```python
from build123d import *

# Parameters (mm, degrees)
SKETCH1_R           = 1.175
BOSS_EXTRUDE1_DEPTH = 6.4
BOSS_EXTRUDE2_DEPTH = 3.2
SKETCH4_W           = 0.5
SKETCH4_H           = 3.9
BOSS_EXTRUDE3_DEPTH = 3.2
SKETCH5_R           = 0.8
CUT_EXTRUDE1_DEPTH  = 22.246411462


with BuildPart() as part:
    # Sketch1 → Boss-Extrude1 (new body)
    with BuildSketch(Plane(origin=(0, 0, 0), x_dir=(1, 0, 0), z_dir=(0, 1, 0))):
        Polygon((-10.95, -2.5), (-10.75, -2.7), (-8.25, -2.7), (-8.05, -2.5), (-1.45, -2.5), (-1.25, -2.7), (1.25, -2.7), (1.45, -2.5), (5.2, -2.5), (5.2, 7), (-4.7, 7), (-5.4, 7.7), (-14.6, 7.7), (-14.6, -2.5), align=None)
        with Locations(Location((0, 0, 0), (0, 0, 270))):
            Circle(SKETCH1_R, mode=Mode.SUBTRACT)
        with Locations(Location((-9.5, 0, 0), (0, 0, 270))):
            Circle(SKETCH1_R, mode=Mode.SUBTRACT)
    extrude(amount=BOSS_EXTRUDE1_DEPTH)

    # Sketch3 → Boss-Extrude2 (add)
    with BuildSketch(Plane(origin=(0, 1.6, 0), x_dir=(1, 0, 0), z_dir=(0, 1, 0))):
        with BuildLine():
            Line((-8.5, 7), (-6.5, 7))
            Line((-6.5, 7), (-6.5, 7.9))
            ThreePointArc((-6.5, 7.9), (-7.5, 8.9), (-8.5, 7.9))
            Line((-8.5, 7.9), (-8.5, 7))
        make_face()
    extrude(amount=BOSS_EXTRUDE2_DEPTH)

    # Sketch4 → Boss-Extrude3 (add)
    with BuildSketch(Plane(origin=(0, 1.6, 0), x_dir=(1, 0, 0), z_dir=(0, 1, 0))):
        with Locations((-12.75, -4.45)):
            Rectangle(SKETCH4_W, SKETCH4_H)
        with Locations((-3.95, -4.45)):
            Rectangle(SKETCH4_W, SKETCH4_H)
        with Locations((3.35, -4.45)):
            Rectangle(SKETCH4_W, SKETCH4_H)
    extrude(amount=BOSS_EXTRUDE3_DEPTH)

    # Sketch5 → Cut-Extrude1 (cut, through all)
    with BuildSketch(Plane(origin=(3.6, 0, 0), x_dir=(0, 0, -1), z_dir=(1, 0, 0))):
        with Locations((-4.8, 3.2)):
            Circle(SKETCH5_R)
    extrude(amount=-CUT_EXTRUDE1_DEPTH, mode=Mode.SUBTRACT)


solid = part.part
```
Work out the finished part from the listing and answer in its coordinate system (mm). A direction names the side the tool comes from. Round coordinates to 2 decimals unless told otherwise and drop trailing zeros. Order: outer loops, then holes, each group sorted by start corner. A loop starts at its lowest first (then second) coordinate and runs counter-clockwise, first axis right, second up.
Q1. Given pin 1 Ø0.6 at (x, z) = (-4, 5) entering from -Y; pin 2 Ø1.2 at (x, y) = (0, 3) entering from +Z; pin 3 Ø1.4 at (y, z) = (3.2, 4.8) entering from -X; pin 4 Ø1.6 at (y, z) = (3, 4.5) entering from +X, each flat-ended and moving along its own axis, determine where each tip first touches the part or whether it passes through.
Solution:
pin 1: stops at y = 1.6
pin 2: stops at z = 2.7
pin 3: passes through
pin 4: stops at x = 3.6
Q2. A cutting plane is placed at B-B, the plane x = 0. Determine the outline of the cut face in (y, z) (3 decimals).
Solution:
outline: (0, -7) - (6.4, -7) - (6.4, -1.175) - (0, -1.175) - close; (0, 1.175) - (6.4, 1.175) - (6.4, 2.7) - (0, 2.7) - close
Q3. A cutting plane is placed at C-C, the plane z = 3.75. Determine the outline of the cut face in (x, y), then the cut area to 3 significant figures.
Solution:
outline: (-13, 1.6) - (-12.5, 1.6) - (-12.5, 4.8) - (-13, 4.8) - close; (-4.2, 1.6) - (-3.7, 1.6) - (-3.7, 4.8) - (-4.2, 4.8) - close; (3.1, 1.6) - (3.6, 1.6) - (3.6, 4.8) - (3.1, 4.8) - close
area: 4.80 mm2
Q4. The mould has two halves that part along Y. Classify faces 1 (the cylindrical face through (-12.747, 3.993, 4.904)), 2 (the flat face through (-8, 1.6, -8)), 3 (the flat face through (-4.2, 4, 4)): pulls with the +Y half, pulls with the -Y half, needs draft (parallel to the pull), parting line crosses it, or undercut.
Solution:
face 1: undercut
face 2: pulls with the -Y half
face 3: needs draft
Q5. Find the intervals of material crossed by line 1 along X through (y, z) = (1.75, 3.25); line 2 along Y through (x, z) = (-12.55, 4.8); line 3 along X through (y, z) = (4.75, 0) (3 decimals), in increasing order.
Solution:
line 1: x = -13 to -12.5, -4.2 to -3.7, 3.1 to 3.6
line 2: y = 1.6 to 2.4, 4 to 4.8
line 3: x = -14.6 to -10.675, -8.325 to -1.175, 1.175 to 5.2
Q6. A cutting plane is placed at D-D, the plane y = 3.2. Count the separate pieces of the cut face and the enclosed holes in it, then the cut area to 3 significant figures.
Solution:
separate pieces: 4
enclosed holes: 2
area: 193 mm2
Q7. A tool of negligible diameter and unlimited length cuts with its end or side. For faces 4 (the flat face through (-10, 3, 2.7)), 5 (the flat face through (-8, 4.8, -8)), 6 (the flat face through (-13, 4, 4)), 7 (the flat face through (0, 3, -7)), from which of +Z, -Z, +X, -X, +Y, -Y can it reach the whole face along a straight path? Write none if from no direction.
Solution:
face 4: +Z, +Y, -Y
face 5: -Z, +X, -X, +Y
face 6: +Z, -X, +Y, -Y
face 7: -Z, +X, +Y, -Y
Q8. A cutting plane is placed at A-A, the plane y = 1. Determine the outline of the cut face in (x, z) (3 decimals), then the cut area to 3 significant figures.
Solution:
outline: (-14.6, -7.7) - (-5.4, -7.7) - (-4.7, -7) - (5.2, -7) - (5.2, 2.5) - (1.45, 2.5) - (1.25, 2.7) - (-1.25, 2.7) - (-1.45, 2.5) - (-8.05, 2.5) - (-8.25, 2.7) - (-10.75, 2.7) - (-10.95, 2.5) - (-14.6, 2.5) - close; hole circle Ø2.35 at (-9.5, 0); hole circle Ø2.35 at (0, 0)
area: 187 mm2
